Work out the finished part from the listing and answer in its coordinate system (mm). Face numbers are marked on the shaded views. A direction names the side the tool comes from. Coordinates: 2 decimals unless noted, no trailing zeros. Write each loop counter-clockwise with the first axis right and the second up, starting at its lowest first coordinate (ties: lowest second). Pieces come first, ordered by that corner, then holes. Notation, with made-up numbers: (-4.75, -33.5) - (32.25, -33.5) arc R11 cw to (32.25, -12.5) - close; hole circle Ø9 at (70.25, -8.5). An arc over 180 degrees is marked (long way). Use a Markdown table: item, result. Add a question column.
(1) The part is cut by section D-D, the plane z = 13. Give the vertices of the cut face in (x, y).
(2) For a pull along Y with two mould halves and no side action, classify the marked faces 3, 4 and 5 as released by +Y, released by -Y, zero draft, split by the parting line, or undercut.
(3) A tool of negligible diameter and unlimited length cuts with its end or side. For the marked faces 1 and 2, from which of +Z, -Z, +X, -X, +Y, -Y can it reach the whole face along a straight path? Write none if from no direction.
(4) The part is cut by section A-A, the plane x = -0.5. Give the vertices of the cut face in (y, z), then the cut area to 3 significant figures.
(5) Given pin 1 Ø1.5 at (x, y) = (-14, 25.5) entering from +Z; pin 2 Ø1.5 at (x, y) = (-13.5, -32.5) entering from -Z; pin 3 Ø1.2 at (x, y) = (19, 25) entering from +Z; pin 4 Ø3 at (y, z) = (-5, 8) entering from -X, each flat-ended and moving along its own axis, determine where each tip first touches the part or whether it passes through.
(6) The part is cut by section B-B, the plane z = 4. Give the vertices of the cut face in (x, y), then the cut area to 3 significant figures.
(7) Find the intervals of material crossed by line 1 (X direction, y = -14.5, z = 9.5); line 2 (Y direction, x = 3, z = 23); line 3 (Y direction, x = -21, z = 15), in increasing order. Write a range as from..to.
(8) The part is cut by section C-C, the plane x = 9.5. Give the vertices of the cut face in (y, z), then the cut area to 3 significant figures.
from build123d import *

# Parameters (mm, degrees)
PAD_DEPTH       = 5
FILLET_R        = 3
PAD001_DEPTH    = 25
SKETCH003_W     = 53
SKETCH003_H     = 16.5
POCKET_DEPTH    = 5
SKETCH001_R     = 2
PAD002_DEPTH    = 4
SKETCH004_R     = 1.05
HOLE_DEPTH      = 6
HOLE_TIPS_R     = 1.05
POCKET001_DEPTH = 10
POCKET002_DEPTH = 5
POCKET003_DEPTH = 5
SKETCH005_R     = 1.05
HOLE001_DEPTH   = 6
HOLE001_TIPS_R  = 1.05


with BuildPart() as part:
    # Sketch → Pad (new body)
    with BuildSketch(Plane.XY):
        with BuildLine():
            Line((-43.5, -34), (43.5, -34))
            ThreePointArc((43.5, -34), (47.035534, -32.535534), (48.5, -29))
            Line((48.5, -29), (48.5, 29))
            ThreePointArc((48.5, 29), (47.035534, 32.535534), (43.5, 34))
            Line((43.5, 34), (-43.5, 34))
            ThreePointArc((-43.5, 34), (-47.035534, 32.535534), (-48.5, 29))
            Line((-48.5, 29), (-48.5, -29))
            ThreePointArc((-48.5, -29), (-47.035534, -32.535534), (-43.5, -34))
        make_face()
    extrude(amount=PAD_DEPTH)

    # Fillet
    fillet_edges = [part.edges().sort_by_distance(p)[0] for p in [
        (0, -34, 0),
        (47.035534, -32.535534, 0),
        (48.5, 0, 0),
        (47.035534, 32.535534, 0),
        (0, 34, 0),
        (-47.035534, 32.535534, 0),
        (-48.5, 0, 0),
        (-47.035534, -32.535534, 0),
    ]]
    fillet(fillet_edges, radius=FILLET_R)

    # Sketch002 (on Face4 of Fillet) → Pad001 (join)
    with BuildSketch(Plane.XY.offset(5)):
        with BuildLine():
            Line((-43.5, -34), (43.5, -34))
            ThreePointArc((43.5, -34), (47.035534, -32.535534), (48.5, -29))
            Line((48.5, -29), (48.5, 29))
            ThreePointArc((48.5, 29), (47.035534, 32.535534), (43.5, 34))
            Line((43.5, 34), (-43.5, 34))
            ThreePointArc((-43.5, 34), (-47.035534, 32.535534), (-48.5, 29))
            Line((-48.5, 29), (-48.5, -29))
            ThreePointArc((-48.5, -29), (-47.035534, -32.535534), (-43.5, -34))
        make_face()
        with BuildLine():
            Line((-39.5, -29), (39.5, -29))
            ThreePointArc((39.5, -29), (43.035534, -27.535534), (44.5, -24))
            Line((44.5, -24), (44.5, 24))
            ThreePointArc((44.5, 24), (43.035534, 27.535534), (39.5, 29))
            Line((39.5, 29), (-39.5, 29))
            ThreePointArc((-39.5, 29), (-43.035534, 27.535534), (-44.5, 24))
            Line((-44.5, 24), (-44.5, -24))
            ThreePointArc((-44.5, -24), (-43.035534, -27.535534), (-39.5, -29))
        make_face(mode=Mode.SUBTRACT)
    extrude(amount=PAD001_DEPTH)

    # Sketch003 (on Face22 of Pad001) → Pocket (cut)
    with BuildSketch(Plane.YZ.offset(48.5)):
        with Locations((0, 18.85)):
            Rectangle(SKETCH003_W, SKETCH003_H)
    extrude(amount=-POCKET_DEPTH, mode=Mode.SUBTRACT)

    # Sketch001 (on Face4 of Fillet) → Pad002 (join)
    with BuildSketch(Plane.XY.offset(5)):
        with Locations((18.99123, 24.5)):
            Circle(SKETCH001_R)
        with Locations((18.99123, -24.5)):
            Circle(SKETCH001_R)
        with Locations((-39.00877, -24.5)):
            Circle(SKETCH001_R)
        with Locations((-39.00877, 24.5)):
            Circle(SKETCH001_R)
    extrude(amount=PAD002_DEPTH)

    # Sketch004 (on Face39 of Pad002) → Hole (cut)
    with BuildSketch(Plane.XY.offset(9)):
        with Locations((-39.00877, 24.5)):
            Circle(SKETCH004_R)
        with Locations((18.99123, 24.5)):
            Circle(SKETCH004_R)
        with Locations((18.99123, -24.5)):
            Circle(SKETCH004_R)
        with Locations((-39.00877, -24.5)):
            Circle(SKETCH004_R)
    extrude(amount=-HOLE_DEPTH, mode=Mode.SUBTRACT)

    # Hole tips → Hole tip 1 section 0
    with BuildSketch(Plane.XY.offset(3), mode=Mode.PRIVATE) as hole_tip_1_s0:
        with Locations((-39.00877, 24.5)):
            Circle(HOLE_TIPS_R)
    loft([hole_tip_1_s0.sketch, Vertex(-39.00877, 24.5, 2.369096)], mode=Mode.SUBTRACT)

    # Hole tips → Hole tip 2 section 0
    with BuildSketch(Plane.XY.offset(3), mode=Mode.PRIVATE) as hole_tip_2_s0:
        with Locations((18.99123, 24.5)):
            Circle(HOLE_TIPS_R)
    loft([hole_tip_2_s0.sketch, Vertex(18.99123, 24.5, 2.369096)], mode=Mode.SUBTRACT)

    # Hole tips → Hole tip 3 section 0
    with BuildSketch(Plane.XY.offset(3), mode=Mode.PRIVATE) as hole_tip_3_s0:
        with Locations((18.99123, -24.5)):
            Circle(HOLE_TIPS_R)
    loft([hole_tip_3_s0.sketch, Vertex(18.99123, -24.5, 2.369096)], mode=Mode.SUBTRACT)

    # Hole tips → Hole tip 4 section 0
    with BuildSketch(Plane.XY.offset(3), mode=Mode.PRIVATE) as hole_tip_4_s0:
        with Locations((-39.00877, -24.5)):
            Circle(HOLE_TIPS_R)
    loft([hole_tip_4_s0.sketch, Vertex(-39.00877, -24.5, 2.369096)], mode=Mode.SUBTRACT)

    # Sketch006 (on Face14 of Hole) → Pocket001 (cut)
    with BuildSketch(Plane(origin=(-48.5, 0, 0), x_dir=(0, -1, 0), z_dir=(-1, 0, 0))):
        with BuildLine():
            Line((-5, -0.312917), (5, -0.312917))
            ThreePointArc((5, -0.312917), (5.707107, -0.020023), (6, 0.687083))
            Line((6, 0.687083), (6, 8.687083))
            ThreePointArc((6, 8.687083), (5.707107, 9.39419), (5, 9.687083))
            Line((5, 9.687083), (-5, 9.687083))
            ThreePointArc((-5, 9.687083), (-5.707107, 9.39419), (-6, 8.687083))
            Line((-6, 8.687083), (-6, 0.687083))
            ThreePointArc((-6, 0.687083), (-5.707107, -0.020023), (-5, -0.312917))
        make_face()
    extrude(amount=-POCKET001_DEPTH, mode=Mode.SUBTRACT)

    # Sketch007 (on Face18 of Pocket001) → Pocket002 (cut)
    with BuildSketch(Plane(origin=(-48.5, 0, 0), x_dir=(0, -1, 0), z_dir=(-1, 0, 0))):
        with BuildLine():
            Line((20.078789, 18.994771), (20.078789, 21))
            ThreePointArc((20.078789, 21), (19.785896, 21.707107), (19.078789, 22))
            Line((19.078789, 22), (-18.921211, 22))
            ThreePointArc((-18.921211, 22), (-19.628318, 21.707107), (-19.921211, 21))
            Line((-19.921211, 21), (-19.921211, 18.99124))
            ThreePointArc((-19.921211, 18.99124), (-19.680243, 18.340186), (-19.07347, 18.002899))
            Line((4.75, 18.002899), (-19.07347, 18.002899))
            ThreePointArc((5.75, 17.002899), (5.457107, 17.710006), (4.75, 18.002899))
            Line((5.75, 12.002899), (5.75, 17.002899))
            ThreePointArc((5.75, 12.002899), (6.042893, 11.295792), (6.75, 11.002899))
            Line((11.75, 11.002899), (6.75, 11.002899))
            ThreePointArc((11.75, 11.002899), (12.457107, 11.295792), (12.75, 12.002899))
            Line((12.75, 17.001614), (12.75, 12.002899))
            ThreePointArc((13.751284, 18.001613), (13.043347, 17.709174), (12.75, 17.001614))
            Line((19.077505, 17.994772), (13.751284, 18.001613))
            ThreePointArc((19.077505, 17.994772), (19.785442, 18.28721), (20.078789, 18.994771))
        make_face()
        with BuildLine():
            Line((-18.890292, 24), (19.109708, 24))
            ThreePointArc((19.109708, 24), (19.816815, 24.292893), (20.109708, 25))
            Line((20.109708, 25), (20.109708, 27))
            ThreePointArc((20.109708, 27), (19.816815, 27.707107), (19.109708, 28))
            Line((19.109708, 28), (-18.890292, 28))
            ThreePointArc((-18.890292, 28), (-19.597398, 27.707107), (-19.890292, 27))
            Line((-19.890292, 27), (-19.890292, 25))
            ThreePointArc((-19.890292, 25), (-19.597398, 24.292893), (-18.890292, 24))
        make_face()
    extrude(amount=-POCKET002_DEPTH, mode=Mode.SUBTRACT)

    # Sketch009 (on Face3 of Pocket002) → Pocket003 (cut)
    with BuildSketch(Plane.XZ.offset(34)):
        with BuildLine():
            Line((-37.00877, 8.15), (0.99123, 8.15))
            ThreePointArc((0.99123, 8.15), (1.698337, 8.442893), (1.99123, 9.15))
            Line((1.99123, 9.15), (1.99123, 15.15))
            ThreePointArc((1.99123, 15.15), (1.698337, 15.857107), (0.99123, 16.15))
            Line((0.99123, 16.15), (-37.00877, 16.15))
            ThreePointArc((-37.00877, 16.15), (-37.715877, 15.857107), (-38.00877, 15.15))
            Line((-38.00877, 15.15), (-38.00877, 9.15))
            ThreePointArc((-38.00877, 9.15), (-37.715877, 8.442893), (-37.00877, 8.15))
        make_face()
    extrude(amount=-POCKET003_DEPTH, mode=Mode.SUBTRACT)

    # Sketch005 (on Face9 of Hole) → Hole001 (cut)
    with BuildSketch(Plane.XY.offset(30)):
        with Locations((-44.535534, -30.035534)):
            Circle(SKETCH005_R)
        with Locations((44.534466, -30.034466)):
            Circle(SKETCH005_R)
        with Locations((44.535534, 30.035534)):
            Circle(SKETCH005_R)
        with Locations((-44.535534, 30.035534)):
            Circle(SKETCH005_R)
    extrude(amount=-HOLE001_DEPTH, mode=Mode.SUBTRACT)

    # Hole001 tips → Hole001 tip 1 section 0
    with BuildSketch(Plane.XY.offset(24), mode=Mode.PRIVATE) as hole001_tip_1_s0:
        with Locations((-44.535534, -30.035534)):
            Circle(HOLE001_TIPS_R)
    loft([hole001_tip_1_s0.sketch, Vertex(-44.535534, -30.035534, 23.369096)], mode=Mode.SUBTRACT)

    # Hole001 tips → Hole001 tip 2 section 0
    with BuildSketch(Plane.XY.offset(24), mode=Mode.PRIVATE) as hole001_tip_2_s0:
        with Locations((44.534466, -30.034466)):
            Circle(HOLE001_TIPS_R)
    loft([hole001_tip_2_s0.sketch, Vertex(44.534466, -30.034466, 23.369096)], mode=Mode.SUBTRACT)

    # Hole001 tips → Hole001 tip 3 section 0
    with BuildSketch(Plane.XY.offset(24), mode=Mode.PRIVATE) as hole001_tip_3_s0:
        with Locations((44.535534, 30.035534)):
            Circle(HOLE001_TIPS_R)
    loft([hole001_tip_3_s0.sketch, Vertex(44.535534, 30.035534, 23.369096)], mode=Mode.SUBTRACT)

    # Hole001 tips → Hole001 tip 4 section 0
    with BuildSketch(Plane.XY.offset(24), mode=Mode.PRIVATE) as hole001_tip_4_s0:
        with Locations((-44.535534, 30.035534)):
            Circle(HOLE001_TIPS_R)
    loft([hole001_tip_4_s0.sketch, Vertex(-44.535534, 30.035534, 23.369096)], mode=Mode.SUBTRACT)


solid = part.part
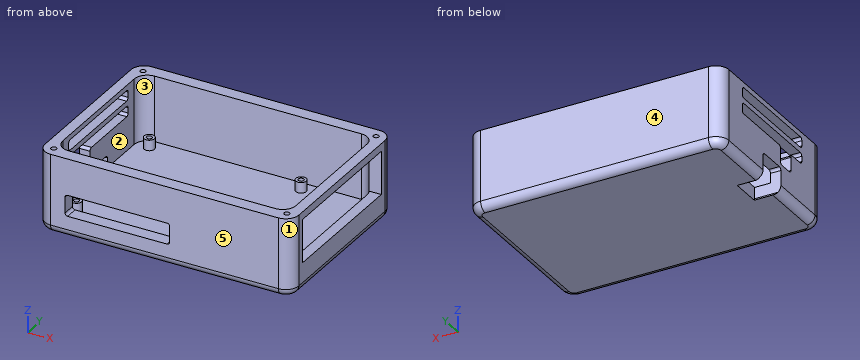
Model answer:
| question | item | result |
|---|---|---|
| 1 | outline | (-48.5, -29) arc R5 ccw to (-43.5, -34) - (-38.01, -34) - (-38.01, -29) - (-39.5, -29) arc R5 cw to (-44.5, -24) - (-44.5, -12.75) - (-48.5, -12.75) - close; (-48.5, -5.75) - (-44.5, -5.75) - (-44.5, 24) arc R5 cw to (-39.5, 29) - (39.5, 29) arc R5 cw to (43.83, 26.5) - (48.5, 26.5) - (48.5, 29) arc R5 ccw to (43.5, 34) - (-43.5, 34) arc R5 ccw to (-48.5, 29) - close; (1.99, -34) - (43.5, -34) arc R5 ccw to (48.5, -29) - (48.5, -26.5) - (43.83, -26.5) arc R5 cw to (39.5, -29) - (1.99, -29) - close |
| 2 | face 3 | undercut |
| 2 | face 4 | released by +Y |
| 2 | face 5 | released by -Y |
| 3 | face 1 | +Z, -Z, +X, -Y |
| 3 | face 2 | +Z |
| 4 | outline | (-34, 3) arc R3 ccw to (-31, 0) - (31, 0) arc R3 ccw to (34, 3) - (34, 30) - (29, 30) - (29, 5) - (-29, 5) - (-29, 8.15) - (-34, 8.15) - close; (-34, 16.15) - (-29, 16.15) - (-29, 30) - (-34, 30) - close |
| 4 | area | 546 mm^2 |
| 5 | pin 1 | z = 5 |
| 5 | pin 2 | z = 0.1 |
| 5 | pin 3 | z = 9 |
| 5 | pin 4 | x = -48.5 |
| 6 | outline | (-48.5, -29) arc R5 ccw to (-43.5, -34) - (43.5, -34) arc R5 ccw to (48.5, -29) - (48.5, 29) arc R5 ccw to (43.5, 34) - (-43.5, 34) arc R5 ccw to (-48.5, 29) - (-48.5, 6) - (-38.5, 6) - (-38.5, -6) - (-48.5, -6) - close; hole circle Ø2.1 at (-39.01, -24.5); hole circle Ø2.1 at (-39.01, 24.5); hole circle Ø2.1 at (18.99, -24.5); hole circle Ø2.1 at (18.99, 24.5) |
| 6 | area | 6,440 mm^2 |
| 7 | line 1 | -48.5..-44.5, 44.5..48.5 |
| 7 | line 2 | -34..-29, 29..34 |
| 7 | line 3 | 29..34 |
| 8 | outline | (-34, 3) arc R3 ccw to (-31, 0) - (31, 0) arc R3 ccw to (34, 3) - (34, 30) - (29, 30) - (29, 5) - (-29, 5) - (-29, 30) - (-34, 30) - close |
| 8 | area | 586 mm^2 |
